Could you check a few things on this model? Use its own coordinates, in mm. Round coordinates to 2 decimals unless told otherwise and drop trailing zeros.
```python
from build123d import *

# Parameters (mm, degrees)
SKETCH1_W           = 359.156
SKETCH1_H           = 127
BOSS_EXTRUDE1_DEPTH = 19.05
CUT_EXTRUDE1_REACH  = 21.05
SKETCH2_R           = 2.85115
CUT_EXTRUDE2_START  = -19.05
SKETCH3_R           = 3.175
CUT_EXTRUDE2_DEPTH  = 6.35


with BuildPart() as part:
    # Sketch1 → Boss-Extrude1 (new body)
    with BuildSketch(Plane.XY):
        with Locations((179.578, 63.5)):
            Rectangle(SKETCH1_W, SKETCH1_H)
    extrude(amount=BOSS_EXTRUDE1_DEPTH)

    # Sketch2 → Cut-Extrude1 (cut, up to next)
    with BuildSketch(Plane.XY.offset(19.05), mode=Mode.PRIVATE) as cut_extrude1_sk1:
        with Locations((48.82515, 82.96275)):
            Circle(SKETCH2_R)
    cut_extrude1_tool1 = extrude(cut_extrude1_sk1.sketch, amount=-CUT_EXTRUDE1_REACH, mode=Mode.PRIVATE) & part.part
    add(cut_extrude1_tool1.solids().sort_by_distance((48.82515, 82.96275, 19.05))[0], mode=Mode.SUBTRACT)
    # Sketch2 → Cut-Extrude1 (cut, up to next)
    with BuildSketch(Plane.XY.offset(19.05), mode=Mode.PRIVATE) as cut_extrude1_sk2:
        with Locations((48.82515, 107.53725)):
            Circle(SKETCH2_R)
    cut_extrude1_tool2 = extrude(cut_extrude1_sk2.sketch, amount=-CUT_EXTRUDE1_REACH, mode=Mode.PRIVATE) & part.part
    add(cut_extrude1_tool2.solids().sort_by_distance((48.82515, 107.53725, 19.05))[0], mode=Mode.SUBTRACT)
    # Sketch2 → Cut-Extrude1 (cut, up to next)
    with BuildSketch(Plane.XY.offset(19.05), mode=Mode.PRIVATE) as cut_extrude1_sk3:
        with Locations((81.47685, 107.53725)):
            Circle(SKETCH2_R)
    cut_extrude1_tool3 = extrude(cut_extrude1_sk3.sketch, amount=-CUT_EXTRUDE1_REACH, mode=Mode.PRIVATE) & part.part
    add(cut_extrude1_tool3.solids().sort_by_distance((81.47685, 107.53725, 19.05))[0], mode=Mode.SUBTRACT)
    # Sketch2 → Cut-Extrude1 (cut, up to next)
    with BuildSketch(Plane.XY.offset(19.05), mode=Mode.PRIVATE) as cut_extrude1_sk4:
        with Locations((81.47685, 82.96275)):
            Circle(SKETCH2_R)
    cut_extrude1_tool4 = extrude(cut_extrude1_sk4.sketch, amount=-CUT_EXTRUDE1_REACH, mode=Mode.PRIVATE) & part.part
    add(cut_extrude1_tool4.solids().sort_by_distance((81.47685, 82.96275, 19.05))[0], mode=Mode.SUBTRACT)

    # Sketch3 → Cut-Extrude2 (cut)
    with BuildSketch(Plane(origin=(0, 0, 0), x_dir=(-1, 0, 0), z_dir=(0, 0, -1)).offset(CUT_EXTRUDE2_START)):
        with Locations((-65.151, 117.475)):
            Circle(SKETCH3_R)
    extrude(amount=CUT_EXTRUDE2_DEPTH, mode=Mode.SUBTRACT)


solid = part.part
```
Q1. For P1, Ø9, axis at x = 48.83, y = 107.54, coming from the -Z side; P2, Ø1.9, axis at x = 66, y = 117, coming from the +Z side, each with a flat end and sliding along its axis, tell me the tip position at first contact or that it passes through.
Q2. I need wall thicknesses on L1, parallel to X at y = 110, z = 15; L2, parallel to X at y = 119.5, z = 15.5. Which ranges of each line are inside material? Lowest first, please.
Q3. We'd pull the mould along X, two halves only. Please class faces 1 (the flat face through (65, 118, 12.7)), 2 (the flat face through (177, 0, 9)), 3 (the cylindrical face through (65.839, 114.376, 15.919)), 4 (the flat face through (359.156, 63, 9)): released by +X, released by -X, zero draft, split by the parting line, or undercut.
Filled in:
1. P1: stops at z = 0
1. P2: stops at z = 12.7
2. L1: x = 0 to 47.39, 50.26 to 80.04, 82.91 to 359.16
2. L2: x = 0 to 62.71, 67.6 to 359.16
3. face 1: undercut
3. face 2: zero draft
3. face 3: undercut
3. face 4: released by +X
